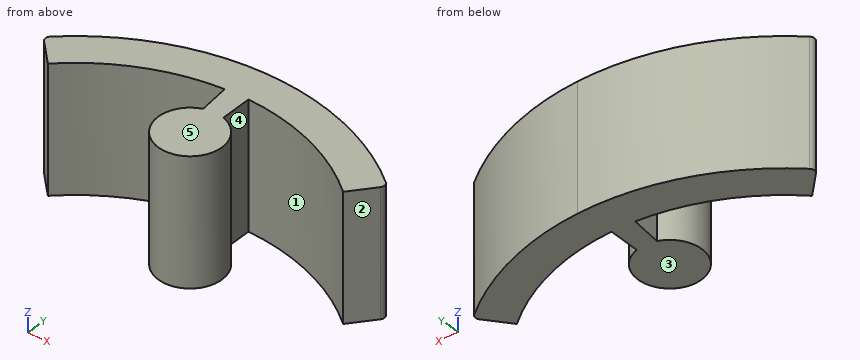
from build123d import *

# Parameters (mm, degrees)
F1_DEPTH = 6


with BuildPart() as f1:
    # F0 (on Top) → F1 (new body)
    with BuildSketch(Plane.XY):
        with BuildLine():
            ThreePointArc((-8.05516, 8.416466), (-8.132287, 8.238597), (-8.059079, 8.059079))
            Line((-8.059079, 8.059079), (-7.071068, 7.071068))
            ThreePointArc((-7.071068, 7.071068), (-4.31807, 9.01966), (-1.073848, 9.942175))
            Line((-1.073848, 9.942175), (-0.918199, 8.50111))
            ThreePointArc((-0.918199, 8.50111), (-0.301868, 5.602173), (-0.000613, 8.550553))
            Line((-0.000613, 8.550553), (-0.000613, 10))
            ThreePointArc((-0.000613, 10), (3.325891, 9.430718), (6.273586, 7.787305))
            Line((6.273586, 7.787305), (7.150168, 8.875393))
            ThreePointArc((7.150168, 8.875393), (7.203741, 9.061715), (7.108018, 9.230308))
            ThreePointArc((7.108018, 9.230308), (3.875, 10.986668), (0.255482, 11.647198))
            ThreePointArc((0.255482, 11.647198), (-4.221155, 10.858377), (-8.05516, 8.416466))
        make_face()
    extrude(amount=F1_DEPTH)


solid = f1.part
Geometry check sheet. Reference: the model listing, model coordinates, mm. Face numbers are marked on the shaded views. A direction names the side the tool comes from. Give positions to 0.01 mm unless a question says otherwise; leave off trailing zeros. Order: outer loops, then holes, each group sorted by start corner. A loop starts at its lowest first (then second) coordinate and runs counter-clockwise, first axis right, second up.
1) Cross-section at C-C (x = 0.5). Record the boundary of the cut face in (y, z).
Results are:
outline: (5.89, 0) - (8.31, 0) - (8.31, 6) - (5.89, 6) - close; (9.99, 0) - (11.64, 0) - (11.64, 6) - (9.99, 6) - close
2) Cross-section at B-B (y = 7.5). Record the boundary of the cut face in (x, z).
Results are:
outline: (-7.5, 0) - (-6.61, 0) - (-6.61, 6) - (-7.5, 6) - close; (-1.83, 0) - (1.06, 0) - (1.06, 6) - (-1.83, 6) - close
3) Cross-section at A-A (z = 4.7). Record the boundary of the cut face in (x, y).
Results are:
outline: (-8.06, 8.06) - (-7.07, 7.07) arc R10 cw to (-1.07, 9.94) - (-0.92, 8.5) arc R1.5 ccw (long way) to (0, 8.55) - (0, 10) arc R10 cw to (6.27, 7.79) - (7.15, 8.88) arc R0.25 ccw to (7.11, 9.23) arc R11.65 ccw to (0.26, 11.65) arc R11.65 ccw to (-8.06, 8.42) arc R0.25 ccw to start
4) Cross-section at D-D (y = 9.5). Record the boundary of the cut face in (x, z), then the cut area to 3 significant figures.
Results are:
outline: (-6.74, 0) - (-3.12, 0) - (-3.12, 6) - (-6.74, 6) - close; (-1.03, 0) - (0, 0) - (0, 6) - (-1.03, 6) - close; (3.12, 0) - (6.74, 0) - (6.74, 6) - (3.12, 6) - close
area: 49.6 mm2
5) Gauge pin test, flat ends, axial feed: pin 1 (2 mm diameter, centred on x = 4.5, y = 9, fed in from -Z); pin 2 (2 mm diameter, centred on y = 10.5, z = 1, fed in from +X); pin 3 (1.5 mm diameter, centred on y = 10, z = 4, fed in from +X). Record the tip position at first contact, or that the pin passes through.
Results are:
pin 1: stops at z = 0
pin 2: stops at x = 6.74
pin 3: stops at x = 7.08
6) Material ranges on probe 1 along X at (y, z) = (8.75, 1.4); probe 2 along X at (y, z) = (9.25, 0.45); probe 3 along Y at (x, z) = (0.5, 0.5), recorded low to high.
Results are:
probe 1: x = -7.69 to -4.84, -0.95 to 0, 4.84 to 7.05
probe 2: x = -7.08 to -3.8, -1 to 0, 3.8 to 7.08
probe 3: y = 5.89 to 8.31, 9.99 to 11.64
7) Tool access check on the marked faces 4 and 5. Record the directions out of +Z, -Z, +X, -X, +Y, -Y that give a thin tool (end or side, any length) a straight path to the whole face; none if there is none.
Results are:
face 4: +Z, -Z
face 5: +Z, +X, -X, +Y, -Y
8) Draft check along Y on the marked faces 1, 2 and 3. Enter one of: released by +Y, released by -Y, zero draft, split by the parting line, or undercut.
Results are:
face 1: undercut
face 2: released by -Y
face 3: zero draft
